Job drawing, mm, ordinate dimensions from the low corner. One solid piece. A direction names the side the tool comes from. Round coordinates to 2 decimals unless told otherwise and drop trailing zeros. Loops run counter-clockwise (first coordinate to the right, second up) from the corner with the lowest first, then second, coordinate; pieces in that order, holes last.
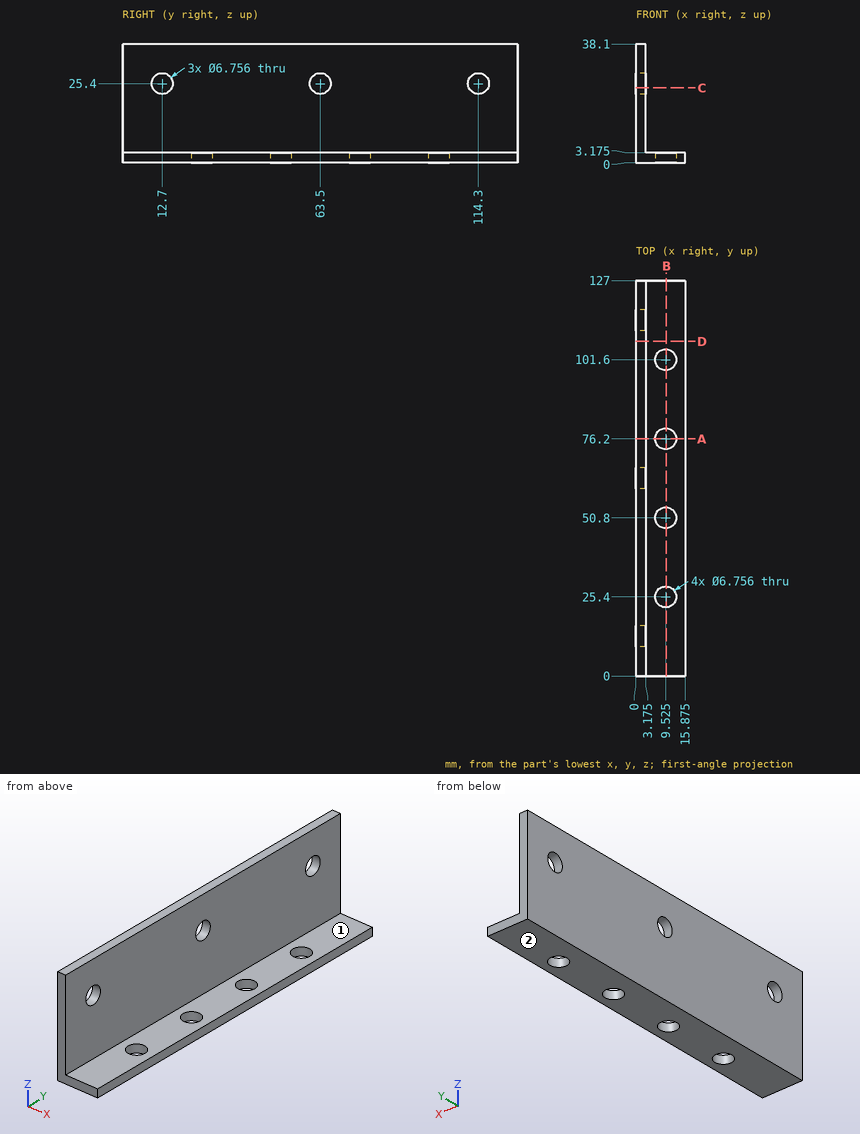
1) Slice it at C-C, the plane z = 24. Give the cut face in (x, y) (1 decimal).
Values:
outline: (0, 0) - (3.2, 0) - (3.2, 9.6) - (0, 9.6) - close; (0, 15.8) - (3.2, 15.8) - (3.2, 60.4) - (0, 60.4) - close; (0, 66.6) - (3.2, 66.6) - (3.2, 111.2) - (0, 111.2) - close; (0, 117.4) - (3.2, 117.4) - (3.2, 127) - (0, 127) - close
2) Wall check: line 1 along Z through (x, y) = (1.2, 12.7); line 2 along Z through (x, y) = (13.5, 40.5) (1 decimal). Give the ranges that are in metal, low to high.
Values:
line 1: z = 0 to 22.02, 28.78 to 38.1
line 2: z = 0 to 3.2
3) Slice it at B-B, the plane x = 9.75. Give the cut face in (y, z) (1 decimal).
Values:
outline: (0, 0) - (22, 0) - (22, 3.2) - (0, 3.2) - close; (28.8, 0) - (47.4, 0) - (47.4, 3.2) - (28.8, 3.2) - close; (54.2, 0) - (72.8, 0) - (72.8, 3.2) - (54.2, 3.2) - close; (79.6, 0) - (98.2, 0) - (98.2, 3.2) - (79.6, 3.2) - close; (105, 0) - (127, 0) - (127, 3.2) - (105, 3.2) - close
4) Drop flat-ended pins along their axis: pin 1 Ø9 at (x, y) = (9.525, 50.8) entering from -Z; pin 2 Ø4 at (x, y) = (8.5, 49.5) entering from +Z (3 decimals); pin 3 Ø1 at (y, z) = (49.5, 15.5) entering from +X (3 decimals). Give the stop position or say it passes through.
Values:
pin 1: stops at z = 0
pin 2: stops at z = 3.175
pin 3: stops at x = 3.175
5) Tool access for the marked faces 1 and 2: list every direction of +Z, -Z, +X, -X, +Y, -Y with a clear straight run to the whole face (end or side of a thin tool).
Values:
face 1: +Z, +X, +Y, -Y
face 2: -Z, +X, -X, +Y, -Y
6) Slice it at A-A, the plane y = 76.2. Give the cut face in (x, z) (1 decimal).
Values:
outline: (0, 0) - (6.1, 0) - (6.1, 3.2) - (3.2, 3.2) - (3.2, 38.1) - (0, 38.1) - close; (12.9, 0) - (15.9, 0) - (15.9, 3.2) - (12.9, 3.2) - close
7) Slice it at D-D, the plane y = 107.5. Give the cut face in (x, z) (1 decimal).
Values:
outline: (0, 0) - (15.9, 0) - (15.9, 3.2) - (3.2, 3.2) - (3.2, 38.1) - (0, 38.1) - close
